Part model, mm, in its own coordinate system. A direction names the side the tool comes from. Coordinates: 2 decimals unless noted, no trailing zeros. Write each loop counter-clockwise with the first axis right and the second up, starting at its lowest first coordinate (ties: lowest second). Pieces come first, ordered by that corner, then holes. Notation, with made-up numbers: (-1, 14) - (5, 14) arc R9 ccw to (5, 28) - close; hole circle Ø6 at (88.25, 73). An arc over 180 degrees is marked (long way). Use a Markdown table: item, result.
Autodesk Inventor part; units mm, degrees
ref_plane "Work Plane1" through (-24, 138, 18) normal (0, 1, 0) x (1, 0, 0)
ref_plane "YZ Plane" through (0, 0, 0) normal (1, 0, 0) x (0, 1, 0)
ref_plane "XZ Plane" through (0, 0, 0) normal (0, 1, 0) x (-1, 0, 0)
sketch "Sketch1" plane through (0, 0, 0) normal (0, 1, 0) x (-1, 0, 0)
  line L0 (90, 60) -> (-90, 60)
  line L1 (-90, 60) -> (-90, -60)
  line L2 (-90, -60) -> (90, -60)
  line L3 (90, -60) -> (90, 60)
  line L4 (90, 60) -> (-90, -60) construction
  line L5 (-90, 60) -> (90, -60) construction
  point P0 (0, 0)
  dimension "d0" = 180
  dimension "d1" = 120
extrude "Extrusion1" add sketch "Sketch1" along normal blind 19
fillet "Fillet1" radius 15 4 edges at (90, 9.5, 60) (90, 9.5, -60) (-90, 9.5, -60) (-90, 9.5, 60)
sketch "Sketch2" plane through (0, 0, 0) normal (0, 0, 1) x (1, 0, 0)
  line L0 (75, 19) -> (-75, 19)
  line L1 (-65, 19) -> (-65, 168)
  arc A0 (65, 168) -> (-65, 168) centre (0, 168) ccw
  line L2 (65, 168) -> (65, 19)
  line L3 (75, 0) -> (-75, 0)
  point P0 (0, 0)
  point P1 (0, 0)
  dimension "d5" = 168
  dimension "d6" = 65
extrude "Extrusion2" add sketch "Sketch2" along normal mid plane 36
sketch "Sketch3" plane through (0, 0, 18) normal (0, 0, 1) x (1, 0, 0)
  arc A0 (65, 168) -> (-65, 168) centre (0, 168) ccw
  arc A1 (24, 142.5245) -> (-24, 142.5245) centre (0, 168) ccw
  arc A2 (-24, 133.4755) -> (24, 133.4755) centre (0, 108) ccw
  line L0 (-24, 142.5245) -> (-24, 133.4755)
  line L1 (24, 142.5245) -> (24, 133.4755)
  point P0 (0, 0)
  dimension "d9" = 70
  dimension "d10" = 70
  dimension "d11" = 60
  dimension "d12" = 48
extrude "Extrusion3" cut sketch "Sketch3" along normal through all both and the other way through all
sketch "Sketch4" plane through (90, 0, 45) normal (1, 0, 0) x (0, 0, -1)
  line L0 (0, 0) -> (90, 0)
  line L1 (15, 0) -> (75, 0)
  line L2 (75, 0) -> (75, 5)
  line L3 (75, 5) -> (15, 5)
  line L4 (15, 5) -> (15, 0)
  line L5 (15, 0) -> (75, 5) construction
  line L6 (75, 0) -> (15, 5) construction
  point P0 (45, 0)
  point P1 (45, 2.5)
  point P2 (45, 0)
  dimension "d15" = 60
  dimension "d16" = 5
extrude "Extrusion4" cut sketch "Sketch4" against normal through all
sketch "Sketch5" plane through (0, 0, 18) normal (0, 0, 1) x (1, 0, 0)
  arc A0 (24, 142.5245) -> (-24, 142.5245) centre (0, 168) ccw
  point P0 (0, 0)
  point P1 (50, 168)
  dimension "d19" = 50
hole "Hole1" at (50, 168, 18) direction (0, 0, -1) diameter 12 end through all counterbore diameter 15 counterbore depth 8
sketch "Sketch6" plane through (0, 0, -18) normal (0, 0, -1) x (-1, 0, 0)
  circle A0 centre (-50, 168) radius 6
  point P0 (0, 0)
hole "Hole2" at (50, 168, -18) direction (0, 0, 1) diameter 15 depth 8
pattern_circular "Circular Pattern1" count 3 over 180 about axis through (0, 168, 18) along (0, 0, 1) of "Hole1", "Hole2"
ref_plane "Work Plane1" through (-24, 138, 18) normal (0, 1, 0) x (1, 0, 0)
mirror "Mirror1" about plane through (-24, 138, 18) normal (0, 1, 0) of "Hole1", "Hole2", "Circular Pattern1"
sketch "Sketch7" plane through (0, 0, 18) normal (0, 0, 1) x (1, 0, 0)
  arc A0 (-24, 133.4755) -> (24, 133.4755) centre (0, 108) ccw
  arc A1 (65, 168) -> (-65, 168) centre (0, 168) ccw
  line L0 (0, 168) -> (35.3553, 203.3553) construction
  line L1 (0, 108) -> (-35.3553, 72.6447) construction
  line L2 (-126, 0) -> (126, 0) construction
  point P0 (0, 0)
  dimension "d37" = 50
  dimension "d38" = 45
hole "Hole3" at (35.3553, 203.3553, 18) at (-35.3553, 72.6447, 18) direction (0, 0, -1) diameter 10 end through all
sketch "Sketch8" plane through (0, 19, 0) normal (0, 1, 0) x (1, 0, 0)
  arc A0 (-90, -45) -> (-75, -60) centre (-75, -45) ccw
  arc A1 (75, -60) -> (90, -45) centre (75, -45) ccw
  arc A2 (90, 45) -> (75, 60) centre (75, 45) ccw
  arc A3 (-75, 60) -> (-90, 45) centre (-75, 45) ccw
  point P0 (0, 0)
hole "Hole4" at (-75, 19, 45) at (75, 19, 45) at (75, 19, -45) at (-75, 19, -45) direction (0, -1, 0) diameter 15 end through all counterbore diameter 20 counterbore depth 13
sketch "Sketch9" plane through (65, 19, 18) normal (1, 0, 0) x (0, 0, -1)
  line L0 (0, 123.5245) -> (36, 123.5245)
  line L1 (36, 114.4755) -> (0, 114.4755)
  line L2 (36, 114.4755) -> (0, 114.4755)
  line L3 (36, 123.5245) -> (0, 114.4755)
  point P0 (18, -19)
  point P1 (18, 119)
  point P2 (18, 119)
hole "Hole5" at (65, 138, 0) direction (-1, 0, 0) diameter 18 depth 41 counterbore diameter 22 counterbore depth 15
mirror "Mirror2" about plane through (0, 0, 0) normal (1, 0, 0) of "Hole5"
ref_plane "Work Plane2" through (-24, 138, 18) normal (0, 1, 0) x (1, 0, 0)
properties part number "Part024. Bearing box" material "Steel, Carbon"
Item 1: Band-saw the part on A-A, the plane z = 5. Count the separate pieces of the cut face and the enclosed holes in it, then the cut area to 3 significant figures.
From the geometry:
| item | result |
|---|---|
| separate pieces | 2 |
| enclosed holes | 8 |
| area | 18,800 mm^2 |
Item 2: Two-plate mould, pull along X, no slides. Class faces 5 (the face through (-0.976, 210.564, 13.944)), 6 (the face through (-36.818, 129.214, 1.951)), 7 (the face through (85.72, 9.63, -55.49)), 8 (the face through (-85.49, 9.63, -55.72)): pulls with the +X half, pulls with the -X half, needs draft (parallel to the pull), parting line crosses it, or undercut.
From the geometry:
| item | result |
|---|---|
| face 5 | undercut |
| face 6 | needs draft |
| face 7 | pulls with the +X half |
| face 8 | pulls with the -X half |
Item 3: Band-saw the part on C-C, the plane x = -17. Give the cut face in (y, z).
From the geometry:
| item | result |
|---|---|
| outline | (0, -60) - (19, -60) - (19, -18) - (77.41, -18) - (77.41, 18) - (19, 18) - (19, 60) - (0, 60) - (0, 30) - (5, 30) - (5, -30) - (0, -30) - close; (198.59, -18) - (230.74, -18) - (230.74, 18) - (198.59, 18) - close |
Item 4: Drill centre lines: probe 1 along Z at (x, y) = (-75, 4.7); probe 2 along X at (y, z) = (108, -11.5); probe 3 along X at (y, z) = (1, 45). Where is each one in solid material? Low to high.
From the geometry:
| item | result |
|---|---|
| probe 1 | -60 to -52.5, -37.5 to -30, 30 to 37.5, 52.5 to 60 |
| probe 2 | -65 to -57.5, -42.5 to -35, 35 to 42.5, 57.5 to 65 |
| probe 3 | -90 to -82.5, -67.5 to 67.5, 82.5 to 90 |
Item 5: Band-saw the part on B-B, the plane z = -40.5. Give the cut face in (x, y).
From the geometry:
| item | result |
|---|---|
| outline | (-90, 0) - (-81, 0) - (-81, 6) - (-83.93, 6) - (-83.93, 19) - (-90, 19) - close; (-69, 0) - (69, 0) - (69, 6) - (66.07, 6) - (66.07, 19) - (-66.07, 19) - (-66.07, 6) - (-69, 6) - close; (81, 0) - (90, 0) - (90, 19) - (83.93, 19) - (83.93, 6) - (81, 6) - close |
Item 6: Which spindle directions (+Z, -Z, +X, -X, +Y, -Y) get a long thin tool onto all of the face, cutting with end or side? Do faces 1 (the face through (1, 3, 30)), 2 (the face through (43.346, 104.539, -13.944)), 3 (the face through (24, 138, 13)), 4 (the face through (68.24, 12.41, 37.63)). Say none if no direction does.
From the geometry:
| item | result |
|---|---|
| face 1 | +X, -X, -Y |
| face 2 | -Z |
| face 3 | +Z, -Z |
| face 4 | +Y |
Item 7: Band-saw the part on D-D, the plane y = 192.5. Give the cut face in (x, z).
From the geometry:
| item | result |
|---|---|
| outline | (-60.21, -18) - (-25, -18) - (-25, 18) - (-60.21, 18) - close; (25, -18) - (60.21, -18) - (60.21, 18) - (25, 18) - close |
Item 8: Drop flat-ended pins along their axis: P1, Ø8, axis at x = 43, y = 134, coming from the +Z side; P2, Ø1.5, axis at x = 6, z = 33.5, coming from the +Y side; P3, Ø16.5, axis at x = -2, y = 59, coming from the -Z side. Give the stop position or say it passes through.
From the geometry:
| item | result |
|---|---|
| P1 | z = 18 |
| P2 | y = 19 |
| P3 | z = -18 |
